from build123d import *

# Parameters (mm, degrees)
SKETCH1_R           = 7.880311683
SKETCH1_R_2         = 1.7907
SKETCH1_R_3         = 4.746605842
BOSS_EXTRUDE1_DEPTH = 12.7
SKETCH5_W           = 7.9375
SKETCH5_H           = 24.448832886
SKETCH5_H_2         = 7.880311683
CUT_EXTRUDE1_DEPTH  = 43.908371508
SKETCH7_R           = 4.7625
BOSS_EXTRUDE3_DEPTH = 9.525


with BuildPart() as part:
    # Sketch1 → Boss-Extrude1 (new body)
    # profile 1 of 4: a face of its own
    with BuildSketch(Plane.XY):
        with Locations((-10.68587239, -26.593250225)):
            Circle(SKETCH1_R)
    # profile 2 of 4: a face of its own
    with BuildSketch(Plane.XY):
        with BuildLine():
            Line((3.60162761, 11.531317118), (-2.805560707, 11.531317118))
            Line((-2.805560707, 11.531317118), (-18.566184073, 11.531317118))
            Line((-18.566184073, 11.531317118), (-18.566184073, -26.593250225))
            ThreePointArc((-18.566184073, -26.593250225), (-10.68587239, -18.712938542), (-2.805560707, -26.593250225))
            Line((-2.805560707, -26.593250225), (-2.805560707, 1.359449775))
            Line((-2.805560707, 1.359449775), (3.60162761, 1.359449775))
            Line((3.60162761, 1.359449775), (3.60162761, 11.531317118))
        make_face()
        with Locations((-10.628684073, -13.868682882)):
            Circle(SKETCH1_R_2, mode=Mode.SUBTRACT)
        with Locations((-5.89797239, 6.451317118)):
            Circle(SKETCH1_R_2, mode=Mode.SUBTRACT)
        with Locations((-0.151184073, 6.451317118)):
            Circle(SKETCH1_R_2, mode=Mode.SUBTRACT)
    # profile 3 of 4: a face of its own
    with BuildSketch(Plane.XY):
        with BuildLine():
            Line((-5.89797239, 27.24757345), (-5.89797239, 28.334249775))
            ThreePointArc((-5.89797239, 28.334249775), (-10.644578231, 23.587643933), (-15.391184073, 28.334249775))
            Line((-15.391184073, 28.334249775), (-15.391184073, 27.2867057))
            ThreePointArc((-15.391184073, 27.2867057), (-15.767187067, 23.64949685), (-16.879292984, 20.16612393))
            Line((-16.879292984, 20.16612393), (-17.078075162, 19.711310306))
            ThreePointArc((-17.078075162, 19.711310306), (-18.190181079, 16.227937386), (-18.566184073, 12.590728536))
            Line((-18.566184073, 12.590728536), (-18.566184073, 11.531317118))
            Line((-18.566184073, 11.531317118), (-2.805560707, 11.531317118))
            Line((-2.805560707, 11.531317118), (-2.805560707, 12.738028185))
            ThreePointArc((-2.805560707, 12.738028185), (-3.176236758, 16.349653807), (-4.272809259, 19.810689652))
            Line((-4.272809259, 19.810689652), (-4.430723837, 20.174911983))
            ThreePointArc((-4.430723837, 20.174911983), (-5.527296339, 23.635947828), (-5.89797239, 27.24757345))
        make_face()
    # profile 4 of 4: a face of its own
    with BuildSketch(Plane.XY):
        with Locations((-10.644578231, 28.334249775)):
            Circle(SKETCH1_R_3)
        with Locations((-10.644578231, 28.334249775)):
            Circle(SKETCH1_R_2, mode=Mode.SUBTRACT)
    extrude(amount=BOSS_EXTRUDE1_DEPTH)

    # Sketch5 → Cut-Extrude1 (cut, through all)
    with BuildSketch(Plane.ZY.offset(18.566184073)):
        with Locations((3.96875, -14.368833782)):
            Rectangle(SKETCH5_W, SKETCH5_H)
        with Locations((3.96875, -30.533406066)):
            Rectangle(SKETCH5_W, SKETCH5_H_2)
        with BuildLine():
            Line((0, -2.144417339), (7.9375, -2.144417339))
            Line((7.9375, -2.144417339), (7.9375, 8.015582661))
            Line((7.9375, 8.015582661), (7.9375, 8.453324113))
            ThreePointArc((7.9375, 8.453324113), (7.673979935, 10.586164901), (6.89926884, 12.590728536))
            Line((6.89926884, 12.590728536), (0, 12.590728536))
            Line((0, 12.590728536), (0, -2.144417339))
        make_face()
        with BuildLine():
            Line((0, 22.08731356), (0, 12.590728536))
            Line((0, 12.590728536), (6.89926884, 12.590728536))
            ThreePointArc((6.89926884, 12.590728536), (5.845775697, 14.135247166), (4.488615022, 15.421132271))
            Line((4.488615022, 15.421132271), (3.372744888, 16.272169226))
            ThreePointArc((3.372744888, 16.272169226), (1.106569634, 18.843459634), (0, 22.08731356))
        make_face()
    extrude(amount=-CUT_EXTRUDE1_DEPTH, mode=Mode.SUBTRACT)

    # Sketch7 → Boss-Extrude3 (add)
    with BuildSketch(Plane(origin=(0, 0, 7.9375), x_dir=(-1, 0, 0), z_dir=(0, 0, -1))):
        with Locations(Location((10.628684073, -26.568682882, 0), (0, 0, 180))):
            Circle(SKETCH7_R)
    extrude(amount=BOSS_EXTRUDE3_DEPTH)


solid = part.part
Geometry check sheet. Reference: the model listing, model coordinates, mm. A direction names the side the tool comes from. Give positions to 0.01 mm unless a question says otherwise; leave off trailing zeros. Loops run counter-clockwise (first coordinate to the right, second up) from the corner with the lowest first, then second, coordinate; pieces in that order, holes last. Notation, with made-up numbers: M 50.5,88.5 L 92.5,88.5 A33 cw 92.5,123.5 Z; hole C 12.5,74.5 d7. An arc over 180 degrees is marked long. Answer as a JSON object with one key per item and string values. Group by question number.
Item 1: Access from +Z, -Z, +X, -X, +Y, -Y to the whole of each face (thin tool, end or side, straight path). Record for faces 5 (the flat face through (0, 11.531, 10)), 6 (the flat face through (-11, 26, 0)), 7 (the flat face through (-10.78, 15.84, 3.94)).
Item 2: Gauge pin test, flat ends, axial feed: pin 1 (1.6 mm diameter, centred on x = -0.5, z = 9, fed in from +Y); pin 2 (4.5 mm diameter, centred on x = -10.64, y = 28.33, fed in from +Z); pin 3 (1.4 mm diameter, centred on y = -7, z = 11, fed in from +X); pin 4 (4 mm diameter, centred on x = -0.15, y = 6.45, fed in from -Z). Record the tip position at first contact, or that the pin passes through.
Item 3: Mould release check, pull along Y, two halves, no side actions. Record for faces 1 (the cylindrical face through (-10.54, 33.08, 6.26)), 2 (the cylindrical face through (-10.78, 18.8, 1.13)), 3 (the flat face through (-10, 0, 12.7)), 4 (the cylindrical face through (-1.47, 7.66, 10.29)): pulls with the +Y half, pulls with the -Y half, needs draft (parallel to the pull), parting line crosses it, or undercut.
Item 4: Sectioned sample at A-A on x = -1.25. Record the boundary of the cut face in (y, z).
Item 5: Sectioned sample at C-C on z = 9.5. Record the boundary of the cut face in (x, y), plus the area to 3 significant figures.
Item 6: Sectioned sample at D-D on y = -29. Record the boundary of the cut face in (x, z), plus the area to 3 significant figures.
Item 7: Sectioned sample at B-B on x = -10. Record the boundary of the cut face in (y, z), plus the area to 3 significant figures.
Item 8: Material ranges on L1, parallel to Y at x = -10.5, z = 11; L2, parallel to X at y = 5, z = 9.75; L3, parallel to Y at x = -10, z = 2.25, recorded low to high.
Findings below:
{
 "1": {"face 5": "+Z, -Z, +X, +Y", "face 6": "-Z, +X, -X, +Y", "face 7": "-Z, +X, -X"},
 "2": {"pin 1": "y = 11.53", "pin 2": "z = 12.7", "pin 3": "x = -2.81", "pin 4": "z = 7.94"},
 "3": {"face 1": "pulls with the +Y half", "face 2": "undercut", "face 3": "needs draft", "face 4": "undercut"},
 "4": {"outline": "M 1.36,7.94 L 5.04,7.94 L 5.04,12.7 L 1.36,12.7 Z; M 7.87,7.94 L 8.45,7.94 A8.76 cw 11.53,7.38 L 11.53,12.7 L 7.87,12.7 Z"},
 "5": {"outline": "M -18.57,-26.59 A7.88 ccw -2.81,-26.59 L -2.81,1.36 L 3.6,1.36 L 3.6,11.53 L -2.81,11.53 L -2.81,12.74 A17.78 ccw -4.27,19.81 L -4.43,20.17 A17.78 cw -5.9,27.25 L -5.9,28.33 A4.75 ccw -15.39,28.33 L -15.39,27.29 A17.78 cw -16.88,20.17 L -17.08,19.71 A17.78 ccw -18.57,12.59 Z; hole C -10.64,28.33 d3.58; hole C -10.63,-13.87 d3.58; hole C -5.9,6.45 d3.58; hole C -0.15,6.45 d3.58", "area": "971 mm2"},
 "6": {"outline": "M -18.19,7.94 L -14.72,7.94 L -14.72,-1.59 L -6.53,-1.59 L -6.53,7.94 L -3.18,7.94 L -3.18,12.7 L -18.19,12.7 Z", "area": "149 mm2"},
 "7": {"outline": "M -34.44,7.94 L -31.29,7.94 L -31.29,-1.59 L -21.85,-1.59 L -21.85,7.94 L -15.55,7.94 L -15.55,12.7 L -34.44,12.7 Z; M -12.19,7.94 L 8.45,7.94 A8.76 cw 15.42,4.49 L 16.27,3.37 A8.76 ccw 22.09,0 L 26.66,0 L 26.66,12.7 L -12.19,12.7 Z; M 30,0 L 33.04,0 L 33.04,12.7 L 30,12.7 Z", "area": "490 mm2"},
 "8": {"L1": "-34.47 to -15.65, -12.08 to 26.55, 30.12 to 33.08", "L2": "-18.57 to -6.95, -4.85 to -1.2, 0.9 to 3.6", "L3": "-31.29 to -21.85, 17.29 to 26.66, 30 to 33.04"}
}
